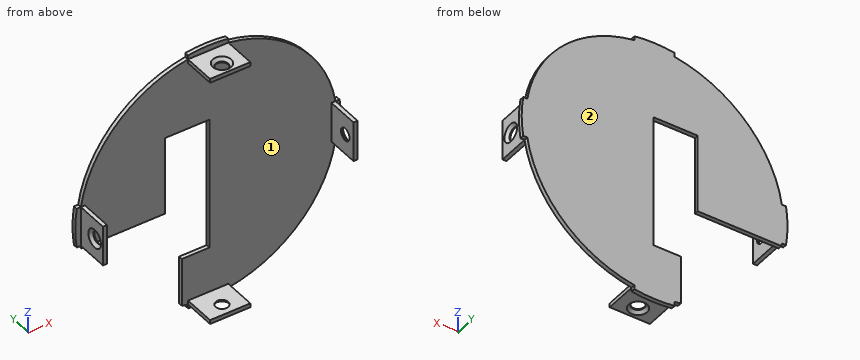
Autodesk Inventor part; units mm, degrees
ref_plane "Work Plane1" through (0, 1, 0) normal (0, 1, 0) x (1, 0, 0)
ref_plane "YZ Plane" through (0, 0, 0) normal (1, 0, 0) x (0, 1, 0)
ref_plane "XZ Plane" through (0, 0, 0) normal (0, 1, 0) x (-1, 0, 0)
sketch "Sketch1" plane through (0, 0, 0) normal (0, 1, 0) x (-1, 0, 0)
  arc A0 (31.6389, 4.7938) -> (6.5, -31.3329) centre (0, 0) ccw
  line L0 (-5, 33) -> (5, 33)
  line L1 (5, 33) -> (5, 31.607)
  line L2 (5, -33) -> (-5, -33)
  line L3 (-5, -33) -> (-5, 5)
  line L4 (-5, 33) -> (5, -33) construction
  line L5 (5, 33) -> (-5, -33) construction
  line L6 (-33, 5) -> (-5, 5)
  line L7 (33, 5) -> (33, -5)
  line L8 (33, -5) -> (31.607, -5)
  line L9 (-33, -5) -> (-33, 5)
  line L10 (-33, 5) -> (33, -5) construction
  line L11 (33, 5) -> (-33, -5) construction
  arc A1 (4.7938, -31.6389) -> (6.5, -31.3329) centre (0, 0) ccw
  line L12 (6.5, -31.3329) -> (6.5, -19.2329)
  line L13 (6.5, -19.2329) -> (-0.3, -19.2329)
  line L14 (-0.3, -19.2329) -> (-0.3, -5.7329)
  line L15 (-0.3, 13.7671) -> (5, 13.7671)
  line L16 (10.7, 13.7671) -> (10.7, 5)
  line L17 (10.7, -5.7329) -> (31.4823, -5.7329)
  arc A2 (31.4823, -5.7329) -> (31.607, -5) centre (0, 0) ccw
  arc A3 (31.6389, -4.7938) -> (31.6389, 4.7938) centre (0, 0) ccw
  line L18 (5, -19.2329) -> (5, -33)
  line L19 (5, 13.7671) -> (5, 5)
  line L20 (10.7, 1.6212) -> (10.7, -5.7329)
  line L21 (-0.3, -5) -> (-0.3, 5)
  arc A4 (6.5, -31.3329) -> (10.7, -30.1581) centre (0, 0) ccw
  line L22 (5, -5) -> (0.7576, -5)
  line L23 (5, 5) -> (10.7, 5)
  line L24 (-5, 5) -> (-0.3, 5)
  line L25 (-5, -5) -> (-33, -5)
  line L26 (-5, 5) -> (-5, 33)
  line L27 (5, 5) -> (5, -5)
  line L28 (5, 31.607) -> (5, 13.7671)
  arc A5 (10.7, -30.1581) -> (31.4823, -5.7329) centre (0, 0) ccw
  arc A6 (6.5, -31.3329) -> (31.6389, -4.7938) centre (0, 0) ccw
  line L29 (-0.3, -5.7329) -> (-0.3, -5)
  line L30 (5, -5) -> (5, -5.7329)
  line L31 (10.7, 5) -> (31.607, 5)
  line L32 (10.7, -5) -> (5, -5)
  line L33 (0.7576, 5) -> (5, 5)
  line L34 (-0.3, 5) -> (0.7576, 5)
  line L35 (5, 13.7671) -> (10.7, 13.7671)
  line L36 (-0.3, 5) -> (-0.3, 13.7671)
  line L37 (31.607, 5) -> (33, 5)
  line L38 (10.7, 5) -> (10.7, 1.6212)
  line L39 (31.607, -5) -> (10.7, -5)
  line L40 (0.7576, -5) -> (-5, -5)
  line L41 (5, -5.7329) -> (5, -19.2329)
  dimension "d0" = 64
  dimension "d1" = 10
  dimension "d2" = 66
  dimension "d3" = 66
  dimension "d4" = 10
  dimension "d11" = 12.1
  dimension "d12" = 6.8
  dimension "d13" = 33
  dimension "d14" = 0.3
  dimension "d15" = 11
  dimension "d16" = 19.5
ref_plane "Work Plane1" through (0, 1, 0) normal (0, 1, 0) x (1, 0, 0)
sketch "Sketch2" plane through (0, 1, 0) normal (0, 1, 0) x (1, 0, 0)
  circle A0 centre (0, 0) radius 33
  dimension "d7" = 66
extrude "Extrusion2" [suppressed]
extrude "Extrusion3" add sketch "Sketch1" along normal blind 1 contours A3 A6 L39 L20 L38 L31 A0 | A0 L37 L7 L8 A6 A3 | L31 L16 L35 L28 A0 | L28 L15 L36 L24 L26 A0 | A0 L26 L0 L1 | A2 L17 L20 L39 | L26 L6 A0 | L6 L3 L25 A0 | A0 L25 L9 L6 | L24 L21 L40 L3 | L25 L3 A0 | L40 L29 L14 L13 L18 A0 L3 | A0 L18 L13 L12 | A0 L18 L2 L3
sketch "Sketch3" plane through (0, 0, 0) normal (0, -1, 0) x (1, 0, 0)
  line L0 (-5, -33) -> (-5, -31.607)
  line L1 (-5, -31.607) -> (5, -31.607)
  line L2 (5, -31.607) -> (5, -30.607)
  line L3 (5, -30.607) -> (-5, -30.607)
  line L4 (-5, -30.607) -> (-5, -31.607)
  line L5 (-33, 5) -> (-31.607, 5)
  line L6 (-31.607, 5) -> (-30.607, 5)
  line L7 (-30.607, 5) -> (-30.607, -5)
  line L8 (-30.607, -5) -> (-31.607, -5)
  line L9 (-31.607, -5) -> (-31.607, 5)
  line L10 (-5, 31.607) -> (-5, 33)
  line L11 (-5, 31.607) -> (5, 31.607)
  line L12 (5, 31.607) -> (5, 30.607)
  line L13 (5, 30.607) -> (-5, 30.607)
  line L14 (-5, 30.607) -> (-5, 31.607)
  line L15 (31.607, 5) -> (30.607, 5)
  line L16 (30.607, 5) -> (30.607, -5)
  line L17 (30.607, -5) -> (31.607, -5)
  line L18 (31.607, -5) -> (31.607, 5)
  line L19 (31.607, 5) -> (33, 5)
  dimension "d21" = 10
  dimension "d22" = 1
  dimension "d23" = 1
  dimension "d24" = 10
  dimension "d25" = 10
  dimension "d26" = 1
  dimension "d27" = 1
  dimension "d28" = 10
extrude "Extrusion4" add sketch "Sketch3" along normal blind 8
sketch "Sketch4" plane through (31.607, 0, 5) normal (1, 0, 0) x (0, 0, -1)
  circle A0 centre (5, -5) radius 2.295
  line L0 (0, 0) -> (10, 0)
  point P0 (5, 0)
  point P1 (5, 0)
  dimension "d31" = 4.59
  dimension "d32" = 5
hole "Hole1" at (31.607, -5, 0) direction (-1, 0, 0) diameter 3.1 end through all countersink diameter 4.59 countersink angle 90
pattern_circular "Circular Pattern1" count 4 over 360 about axis through (0, 0, 0) along (0, 1, 0) of "Hole1"
sketch "Sketch5" plane through (0, 1, 0) normal (0, 1, 0) x (1, 0, 0)
  circle A0 centre (0, 0) radius 33
  dimension "d43" = 66
extrude "Extrusion5" cut sketch "Sketch5" against normal blind 100 keep common part
properties part number "Hull_top"
The model under review builds one solid part; all positions refer to its coordinate system, in mm. Face numbers are marked on the shaded views. Give positions to 0.01 mm unless a question says otherwise; leave off trailing zeros. Loops run counter-clockwise (first coordinate to the right, second up) from the corner with the lowest first, then second, coordinate; pieces in that order, holes last. Notation, with made-up numbers: (1.5, 30.25) -> (36.5, 30.25) arc R21 ccw to (36.5, 48.25) -> close; hole circle Ø3 at (45.25, -35.5). An arc over 180 degrees is marked (long way). Put each result on its own line as item: value. Start each with the question number.
1. We need section C-C on x = -4. State the section outline as (y, z) points, then the cut area to 3 significant figures.
2. Mouldability with a two-part tool opening along Z and no side actions: class the marked faces 1 and 2 as released by +Z, released by -Z, zero draft, split by the parting line, or undercut.
3. Clearance check with flat-ended pins moving along their axes: P1, Ø5, axis at x = 1.5, y = -6, coming from the +Z side; P2, Ø0.5, axis at x = -31, y = -3, coming from the +Z side; P3, Ø0.7, axis at x = -32, z = -2.5, coming from the -Y side; P4, Ø0.6, axis at y = -3.5, z = -32, coming from the -X side. State where each tip first meets the part, or that it passes through.
4. We need section A-A on z = 0. State the section outline as (x, y) points (3 decimals).
5. Wall thickness on probe 1 along X at (y, z) = (-2.5, 1); probe 2 along Y at (x, z) = (-30.7, 0): over which ranges is each line inside the solid? List them lowest first.
6. We need section B-B on y = -1.5. State the section outline as (x, z) points.
7. We need section D-D on y = -5. State how many separate pieces and enclosed holes the cut face has, then the cut area to 3 significant figures.
Determined:
1. outline: (-8, -31.61) -> (0, -31.61) -> (0, -32.76) -> (1, -32.76) -> (1, -19.23) -> (0, -19.23) -> (0, -30.61) -> (-8, -30.61) -> close; (-8, 30.61) -> (0, 30.61) -> (0, 13.77) -> (1, 13.77) -> (1, 32.76) -> (0, 32.76) -> (0, 31.61) -> (-8, 31.61) -> close
1. area: 48.5 mm^2
2. face 1: undercut
2. face 2: zero draft
3. P1: z = 31.61
3. P2: z = 5
3. P3: y = 0
3. P4: through
4. outline: (-33, 0) -> (-31.607, 0) -> (-31.607, -2.705) -> (-30.862, -3.45) -> (-30.607, -3.45) -> (-30.607, 0) -> (-10.7, 0) -> (-10.7, 1) -> (-33, 1) -> close; (-31.607, -8) -> (-30.607, -8) -> (-30.607, -6.55) -> (-30.862, -6.55) -> (-31.607, -7.295) -> close; (0.3, 0) -> (30.607, 0) -> (30.607, -3.45) -> (30.862, -3.45) -> (31.607, -2.705) -> (31.607, 0) -> (33, 0) -> (33, 1) -> (0.3, 1) -> close; (30.607, -8) -> (31.607, -8) -> (31.607, -7.295) -> (30.862, -6.55) -> (30.607, -6.55) -> close
5. probe 1: -31.61 to -30.61, 30.61 to 31.61
5. probe 2: -8 to -6.55, -3.45 to 1
6. outline: (-31.61, -5) -> (-30.61, -5) -> (-30.61, 5) -> (-31.61, 5) -> close; (-5, -31.61) -> (5, -31.61) -> (5, -30.61) -> (-5, -30.61) -> close; (-5, 30.61) -> (5, 30.61) -> (5, 31.61) -> (-5, 31.61) -> close; (30.61, -5) -> (31.61, -5) -> (31.61, 5) -> (30.61, 5) -> close
7. separate pieces: 8
7. enclosed holes: 0
7. area: 25.4 mm^2
